Read the model definition and answer for the solid it produces. Units are mm, in the model's axes. A direction names the side the tool comes from. Coordinates: 2 decimals unless noted, no trailing zeros. Order: outer loops, then holes, each group sorted by start corner. A loop starts at its lowest first (then second) coordinate and runs counter-clockwise, first axis right, second up. Notation, with made-up numbers: (74, 7.25) -> (96, 7.25) arc R25 cw to (96, 42.25) -> close; hole circle Ø5 at (65, 25). An arc over 180 degrees is marked (long way). Answer as a JSON object with one key per item and string values. Group by question number.
1) Consider L1, parallel to X at y = 54.5, z = -4.25; L2, parallel to Z at x = 0.25, y = 69.5. Determine where each line is inside the solid, lowest interval first.
2) Section A-A on y = 55 is taken. Determine the outline of the cut face in (x, z).
3) Given pin 1 (1.5 mm diameter, centred on y = 85, z = -1, fed in from -X); pin 2 (4 mm diameter, centred on x = -2.5, y = 48, fed in from +Z); pin 3 (1.6 mm diameter, centred on x = -0.5, y = 93.5, fed in from -Z), each flat-ended and moving along its own axis, determine where each tip first touches the part or whether it passes through.
4) Determine the mould class of faces 3 (the flat face through (0, 85, -4)), 4 (the cylindrical face through (-4.88, 44.44, -1.08)), 5 (the flat face through (0, 93, -3.45)) for opening direction Z: released by +Z, released by -Z, zero draft, split by the parting line, or undercut.
5) A tool of negligible diameter and unlimited length cuts with its end or side. For faces 1 (the cylindrical face through (0.151, 92.124, 4.347)), 2 (the conical face through (0, 1, -1)), from which of +Z, -Z, +X, -X, +Y, -Y can it reach the whole face along a straight path? Write none if from no direction.
from build123d import *

# Parameters (mm, degrees)
SKETCH1_R           = 5
BOSS_EXTRUDE1_DEPTH = 85
CHAMFER1_SIZE       = 5
BOSS_EXTRUDE2_DEPTH = 16.45


with BuildPart() as part:
    # Sketch1 → Boss-Extrude1 (new body)
    with BuildSketch(Plane(origin=(0, 0, 0), x_dir=(1, 0, 0), z_dir=(0, 1, 0))):
        with Locations(Location((0, 0, 0), (0, 0, 270))):
            Circle(SKETCH1_R)
    extrude(amount=BOSS_EXTRUDE1_DEPTH)

    # Chamfer1
    chamfer1_edges = [part.edges().sort_by_distance(p)[0] for p in [
        (0, 0, -5),
    ]]
    chamfer(chamfer1_edges, length=CHAMFER1_SIZE)

    # Sketch2 → Boss-Extrude2 (add)
    with BuildSketch(Plane(origin=(0, 85, 0), x_dir=(1, 0, 0), z_dir=(0, 1, 0))):
        with BuildLine():
            Line((-2.64952826, 3.45), (2.64952826, 3.45))
            ThreePointArc((2.64952826, 3.45), (0, -4.35), (-2.64952826, 3.45))
        make_face()
    extrude(amount=BOSS_EXTRUDE2_DEPTH)

    # Chamfer2: read off the stored shape, not the designer's step
    # Chamfer2 outline → Chamfer2 (revolve, cut)
    with BuildSketch(Plane.XY):
        Polygon((4.35, 101.45), (2.35, 101.45), (4.35, 99.45), align=None)
    revolve(axis=Axis((0, 0, 0), (0, 1, 0)), mode=Mode.SUBTRACT)

    # Sketch3 → Cut-Revolve1 (revolve, cut)
    with BuildSketch(Plane(origin=(0, 0, 0), x_dir=(0, 0, -1), z_dir=(1, 0, 0))):
        with BuildLine():
            Line((-4.35, 91.2), (-4.35, 91.7))
            ThreePointArc((-4.35, 91.7), (-4.1, 91.45), (-4.35, 91.2))
        make_face()
    revolve(axis=Axis((0, 91.2, 4.35), (0, 1, 0)), mode=Mode.SUBTRACT)


solid = part.part
Worked answers:
{
 "1": {"L1": "x = -2.63 to 2.63", "L2": "z = -4.99 to 4.99"},
 "2": {"outline": "circle Ø10 at (0, 0)"},
 "3": {"pin 1": "stops at x = -4.99", "pin 2": "stops at z = 4.97", "pin 3": "stops at z = -3.45"},
 "4": {"face 3": "zero draft", "face 4": "split by the parting line", "face 5": "released by -Z"},
 "5": {"face 1": "+Y", "face 2": "-Y"}
}
